Autodesk Inventor part; units mm, degrees
ref_plane "YZ Plane" through (0, 0, 0) normal (1, 0, 0) x (0, 1, 0)
ref_plane "XZ Plane" through (0, 0, 0) normal (0, 1, 0) x (-1, 0, 0)
ref_plane "XY Plane" through (0, 0, 0) normal (0, 0, 1) x (1, 0, 0)
sketch "Sketch1" plane through (0, 0, 0) normal (0, 1, 0) x (-1, 0, 0)
  line L0 (-2.1276, -24.9093) -> (-2.0134, -30.0178)
  line L1 (1.9856, -29.9284) -> (1.8739, -24.9297)
  arc A0 (-2.0134, -30.0178) -> (1.9856, -29.9284) centre (-0.0139, -29.9731) ccw
  arc A1 (-12.1587, -27.5189) -> (-8.3703, -28.8026) centre (-10.2645, -28.1608) ccw
  line L2 (-8.3703, -28.8026) -> (-6.7656, -24.0671)
  line L3 (-10.5187, -22.6794) -> (-12.1587, -27.5189)
  arc A2 (-20.8374, -21.7008) -> (-17.7166, -24.2028) centre (-19.277, -22.9518) ccw
  line L4 (-17.7166, -24.2028) -> (-14.589, -20.3017)
  line L5 (-17.6412, -17.7141) -> (-20.8374, -21.7008)
  arc A3 (-27.0029, -13.2653) -> (-24.926, -16.6838) centre (-25.9644, -14.9745) ccw
  line L6 (-24.926, -16.6838) -> (-20.6528, -14.0877)
  line L7 (-22.6359, -10.6121) -> (-27.0029, -13.2653)
  arc A4 (-29.9114, -3.2297) -> (-29.1289, -7.1525) centre (-29.5202, -5.1911) ccw
  line L8 (-29.1289, -7.1525) -> (-24.2255, -6.1744)
  line L9 (-24.9003, -2.2302) -> (-29.9114, -3.2297)
  arc A5 (-29.2121, 7.1953) -> (-29.8185, 3.2416) centre (-29.5153, 5.2185) ccw
  line L10 (-29.8185, 3.2416) -> (-24.8763, 2.4836)
  line L11 (-24.1614, 6.4207) -> (-29.2121, 7.1953)
  arc A6 (-24.9895, 16.7526) -> (-26.9116, 13.2446) centre (-25.9505, 14.9986) ccw
  line L12 (-26.9116, 13.2446) -> (-22.5267, 10.842)
  line L13 (-20.5083, 14.2972) -> (-24.9895, 16.7526)
  arc A7 (-17.7527, 24.2892) -> (-20.7587, 21.6502) centre (-19.2557, 22.9697) ccw
  line L14 (-20.7587, 21.6502) -> (-17.46, 17.8927)
  line L15 (-14.3816, 20.4492) -> (-17.7527, 24.2892)
  arc A8 (-8.3747, 28.8961) -> (-12.102, 27.4444) centre (-10.2384, 28.1703) ccw
  line L16 (-12.102, 27.4444) -> (-10.2873, 22.7853)
  line L17 (-6.5202, 24.1348) -> (-8.3747, 28.8961)
  arc A9 (2.0134, 30.0178) -> (-1.9856, 29.9284) centre (0.0139, 29.9731) ccw
  line L18 (-1.9856, 29.9284) -> (-1.8739, 24.9297)
  line L19 (2.1276, 24.9093) -> (2.0134, 30.0178)
  arc A10 (1.8739, -24.9297) -> (24.6616, 4.0993) centre (0, 0) ccw
  circle A11 centre (52.9459, 46.5257) radius 5
  line L20 (45.8748, 53.5968) -> (13.3899, 21.1118)
  line L21 (24.6616, 4.0993) -> (60.017, 39.4546)
  arc A12 (60.017, 39.4546) -> (45.8748, 53.5968) centre (52.9459, 46.5257) ccw
  arc A13 (13.3899, 21.1118) -> (2.1276, 24.9093) centre (0, 0) ccw
  arc A14 (-1.8739, 24.9297) -> (-6.5202, 24.1348) centre (0, 0) ccw
  arc A15 (-10.2873, 22.7853) -> (-14.3816, 20.4492) centre (0, 0) ccw
  arc A16 (-17.46, 17.8927) -> (-20.5083, 14.2972) centre (0, 0) ccw
  arc A17 (-22.5267, 10.842) -> (-24.1614, 6.4207) centre (0, 0) ccw
  arc A18 (-24.8763, 2.4836) -> (-24.9003, -2.2302) centre (0, 0) ccw
  arc A19 (-24.2255, -6.1744) -> (-22.6359, -10.6121) centre (0, 0) ccw
  arc A20 (-20.6528, -14.0877) -> (-17.6412, -17.7141) centre (0, 0) ccw
  arc A21 (-14.589, -20.3017) -> (-10.5187, -22.6794) centre (0, 0) ccw
  arc A22 (-6.7656, -24.0671) -> (-2.1276, -24.9093) centre (0, 0) ccw
  circle A23 centre (0, 0) radius 5
  point P0 (28.2843, 28.2843)
  dimension "d9" = 180
  dimension "d17" = 10
  dimension "d18" = 10
  dimension "d19" = 20
  dimension "d20" = 25
  dimension "d21" = 5
  dimension "d22" = 2
  dimension "d23" = 50
extrude "Extrusion1" add sketch "Sketch1" along normal blind 5
properties part number "gerigi"
CAD build for the part. Positions are in the model's coordinates, mm. A direction names the side the tool comes from. Give positions to 0.01 mm unless a question says otherwise; leave off trailing zeros. Loops run counter-clockwise (first coordinate to the right, second up) from the corner with the lowest first, then second, coordinate; pieces in that order, holes last. Notation, with made-up numbers: M -9,-36 L 13,-36 A29 ccw 13,-4 Z; hole C 87.25,39 d2. An arc over 180 degrees is marked long. Answer in a Markdown table with one row per item. Add a question column.
Item 1: Band-saw the part on D-D on y = 2.75. Give the number of separate pieces and of enclosed holes in the cut face, then the cut area to 3 significant figures.
Item 2: Band-saw the part on A-A on z = 0. Give the cut face in (x, y), then the cut area to 3 significant figures.
Item 3: Probe probe 1 along X at (y, z) = (0.5, 29); probe 2 along Z at (x, y) = (0, 1.6); probe 3 along X at (y, z) = (3.35, 28.5). List the from-to ranges inside material, lowest first.
Item 4: Tool access for faces 1 (the face through (16.04, 2.46, 22.34)), 2 (the face through (23.524, 2.465, -8.462)), 3 (the face through (4.434, 2.465, -24.604)): list every direction of +Z, -Z, +X, -X, +Y, -Y with a clear straight run to the whole face (end or side of a thin tool).
Item 5: Band-saw the part on C-C on x = -17. Give the cut face in (y, z), then the cut area to 3 significant figures.
Item 6: Band-saw the part on B-B on x = 0. Give the cut face in (y, z).
Item 7: Drop flat-ended pins along their axis: P1, Ø1.5, axis at x = 3, z = 1, coming from the -Y side; P2, Ø1, axis at x = -17.5, y = 4.5, coming from the -Z side; P3, Ø1, axis at y = 3.5, z = -14.5, coming from the +X side; P4, Ø1, axis at x = -36.5, y = 2, coming from the +Z side. Give the stop position or say it passes through.
Item 8: Mould opens along X. For faces 4 (the face through (-59.86, 2.46, 53.75)), 5 (the face through (-15, 0, 13)), 6 (the face through (-29.86, 2.46, 37.58)) say: +X half, -X half, draft (parallel to the pull), parting line (faces both ways), or undercut.
Reply:
| question | item | result |
|---|---|---|
| 1 | separate pieces | 1 |
| 1 | enclosed holes | 2 |
| 1 | area | 3,160 mm^2 |
| 2 | outline | M -25,0 L -5,0 L -5,5 L -25,5 Z; M 5,0 L 25,0 L 25,5 L 5,5 Z |
| 2 | area | 200 mm^2 |
| 3 | probe 1 | x = -49.56 to -21.28, -2.04 to 1.96, 8.42 to 12.06 |
| 3 | probe 2 | z = -31.97 to -5, 5 to 31.97 |
| 3 | probe 3 | x = -49.06 to -20.78, -2.05 to 1.95, 8.22 to 12.21 |
| 4 | face 1 | +Z, +Y, -Y |
| 4 | face 2 | +Y, -Y |
| 4 | face 3 | -Z, +Y, -Y |
| 5 | outline | M 0,-18.33 L 5,-18.33 L 5,24.72 L 0,24.72 Z |
| 5 | area | 215 mm^2 |
| 6 | outline | M 0,-31.97 L 5,-31.97 L 5,-5 L 0,-5 Z; M 0,5 L 5,5 L 5,31.97 L 0,31.97 Z |
| 7 | P1 | passes through |
| 7 | P2 | stops at z = -18.33 |
| 7 | P3 | stops at x = 27.96 |
| 7 | P4 | stops at z = 44.72 |
| 8 | face 4 | parting line |
| 8 | face 5 | draft |
| 8 | face 6 | undercut |
